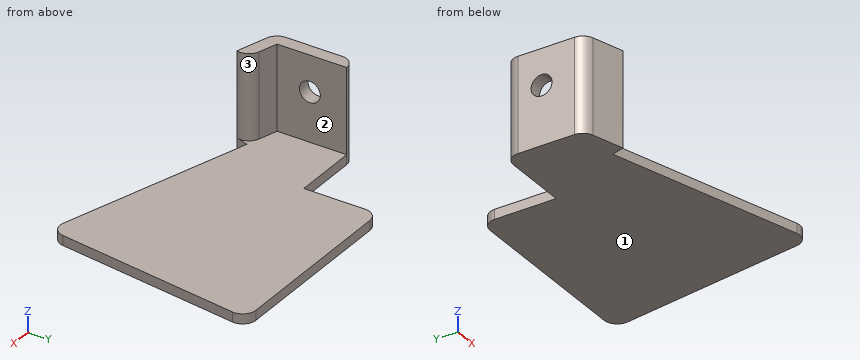
```python
from build123d import *

# Parameters (mm, degrees)
BOSS_EXTRUDE1_DEPTH = 1.5
BOSS_EXTRUDE4_DEPTH = 14.5
FILLET3_R           = 2
CUT_EXTRUDE1_REACH  = 58.101
SKETCH7_R           = 1.6


with BuildPart() as part:
    # Sketch1 → Boss-Extrude1 (new body)
    with BuildSketch(Plane.XY):
        Polygon((-6.174224551, -3.411681894), (24.72754499, -3.411681894), (20.077965687, -36.495157687), (-18.174224551, -24.800289498), (-18.174224551, -14.800289498), (-6.174224551, -14.800289498), align=None)
    extrude(amount=BOSS_EXTRUDE1_DEPTH)

    # Sketch6 → Boss-Extrude4 (add)
    with BuildSketch(Plane(origin=(0, 0, 0), x_dir=(-1, 0, 0), z_dir=(0, 0, -1))):
        Polygon((16.174224551, -25.411750861), (11.392700771, -26.873609384), (11.977444181, -28.786218896), (18.174224551, -26.891673011), (18.174224551, -14.800289498), (16.174224551, -14.800289498), align=None)
    extrude(amount=-BOSS_EXTRUDE4_DEPTH)

    # Fillet3
    fillet3_edges = [part.edges().sort_by_distance(p)[0] for p in [
        (-18.174224551, -26.891673011, 7.25),
        (20.077965687, -36.495157687, 0.75),
        (-6.174224551, -3.411681894, 0.75),
        (24.72754499, -3.411681894, 0.75),
        (-11.392700771, -26.873609384, 8),
        (-18.174224551, -14.800289498, 7.25),
    ]]
    fillet(fillet3_edges, radius=FILLET3_R - 0.0001)  # a hair under: the kernel refuses the full size

    # Sketch7 → Cut-Extrude1 (cut, up to next)
    with BuildSketch(Plane(origin=(-16.174224551, 0, 0), x_dir=(0, 0, -1), z_dir=(1, 0, 0)), mode=Mode.PRIVATE) as cut_extrude1_sk1:
        with Locations((-9, -20.411750861)):
            Circle(SKETCH7_R)
    cut_extrude1_tool1 = extrude(cut_extrude1_sk1.sketch, amount=-CUT_EXTRUDE1_REACH, mode=Mode.PRIVATE) & part.part
    add(cut_extrude1_tool1.solids().sort_by_distance((-16.174225, -20.411751, 9))[0], mode=Mode.SUBTRACT)


solid = part.part
```
Could you check a few things on this model? Use its own coordinates, in mm. Face numbers are marked on the shaded views. A direction names the side the tool comes from. Round coordinates to 2 decimals unless told otherwise and drop trailing zeros. Write each loop counter-clockwise with the first axis right and the second up, starting at its lowest first coordinate (ties: lowest second). Pieces come first, ordered by that corner, then holes.
(1) For pin 1 (6 mm diameter, centred on y = -30, z = 10, fed in from +X); pin 2 (8 mm diameter, centred on y = -9.5, z = 11, fed in from -X); pin 3 (5 mm diameter, centred on y = -20.41, z = 9, fed in from +X); pin 4 (3 mm diameter, centred on x = -13, z = 4.5, fed in from +Y), each with a flat end and sliding along its axis, tell me the tip position at first contact or that it passes through.
Findings below:
pin 1: stops at x = -11.89
pin 2: passes through
pin 3: stops at x = -16.17
pin 4: stops at y = -25.92
(2) Suppose I cut it at D-D on x = 10. Write out the boundary of the cut face in (y, z).
Findings below:
outline: (-33.41, 0) - (-3.41, 0) - (-3.41, 1.5) - (-33.41, 1.5) - close
(3) Which directions (+Z, -Z, +X, -X, +Y, -Y) give clear straight access to the entire face, cutting with the end or side of a thin tool? Please do the marked faces 1, 2 and 3.
Findings below:
face 1: -Z, +X, -X, +Y, -Y
face 2: +Z, +X, +Y
face 3: +Z, +X
(4) If I drill on probe 1 along X at (y, z) = (-23.5, 10.25); probe 2 along Z at (x, y) = (2, -14); probe 3 along Y at (x, z) = (-17.5, 9), over which ranges is the centre line in solid material (lowest first)?
Findings below:
probe 1: x = -18.17 to -16.17
probe 2: z = 0 to 1.5
probe 3: y = -26.91 to -22.01, -18.81 to -15.3
(5) Suppose I cut it at C-C on z = 1. Write out the boundary of the cut face in (x, y).
Findings below:
outline: (-18.17, -25.41) arc R2 ccw to (-16.76, -27.32) - (-11.98, -28.79) - (-11.39, -26.87) - (17.84, -35.81) arc R2 ccw to (20.4, -34.18) - (24.41, -5.69) arc R2 ccw to (22.43, -3.41) - (-4.17, -3.41) arc R2 ccw to (-6.17, -5.41) - (-6.17, -14.8) - (-16.17, -14.8) arc R2 ccw to (-18.17, -16.8) - close
(6) Suppose I cut it at B-B on y = -17.5. Write out the boundary of the cut face in (x, z), and give its area (3 significant figures).
Findings below:
outline: (-18.17, 0) - (22.75, 0) - (22.75, 1.5) - (-16.17, 1.5) - (-16.17, 14.5) - (-18.17, 14.5) - close
area: 87.4 mm2
